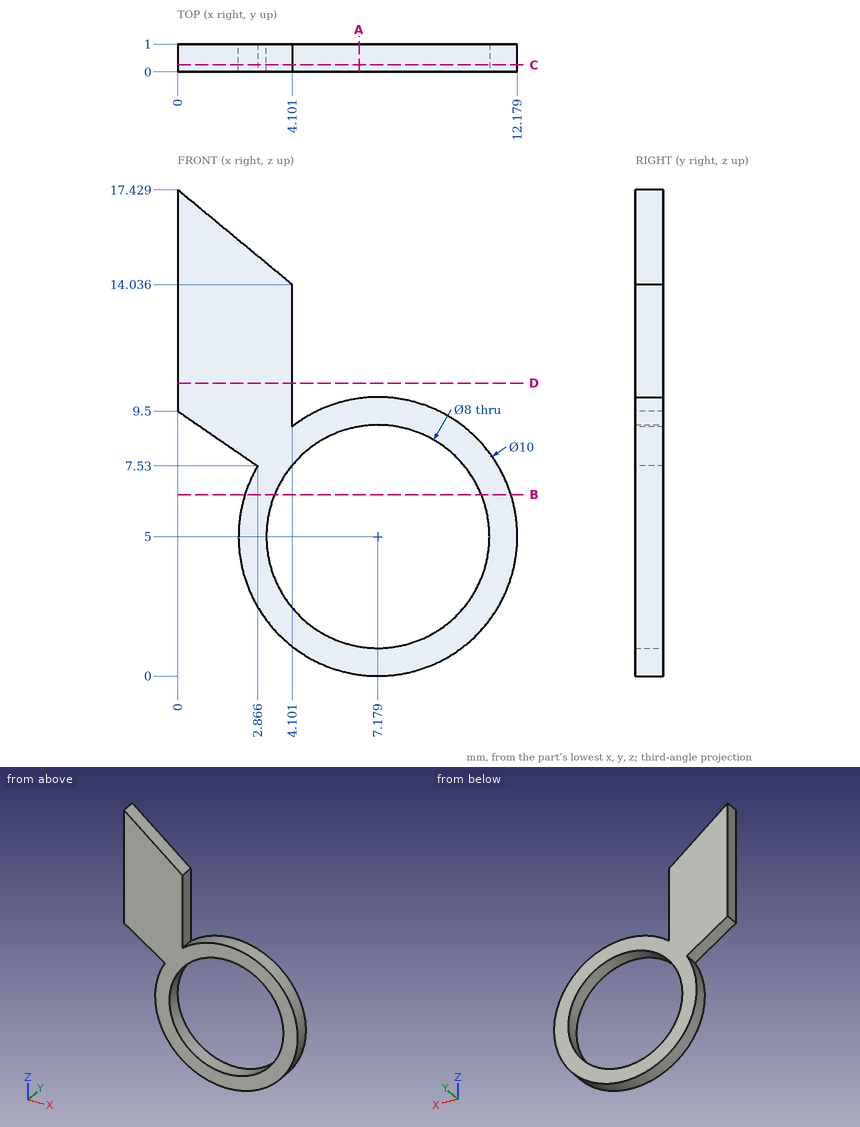
The drawing under review shows one solid part. Ordinate dimensions are in mm from its lowest x, y, z. Coordinates: 2 decimals unless noted, no trailing zeros. Order: outer loops, then holes, each group sorted by start corner. A loop starts at its lowest first (then second) coordinate and runs counter-clockwise, first axis right, second up. Notation, with made-up numbers: (-18, 22.5) - (-5, 22.5) arc R22 cw to (-5, 59.5) - close; hole circle Ø11 at (35, 78). An arc over 180 degrees is marked (long way). Put each result on its own line as item: value.
1) Take a section at D-D, the plane z = 10.5. Give the boundary of the cut face in (x, y).
Response values:
outline: (0, 0) - (4.1, 0) - (4.1, 1) - (0, 1) - close
2) Take a section at B-B, the plane z = 6.5. Give the boundary of the cut face in (x, y).
Response values:
outline: (2.41, 0) - (3.47, 0) - (3.47, 1) - (2.41, 1) - close; (10.89, 0) - (11.95, 0) - (11.95, 1) - (10.89, 1) - close
3) Insertion check: P1, Ø1, axis at x = 1.5, z = 5, coming from the +Y side. The pin has a flat end and moves straight along its axis. Give the tip position at first contact, or say it passes through.
Response values:
P1: passes through
4) Wall thickness on L1, parallel to Z at x = 7, y = 0.1; L2, parallel to Z at x = 4, y = 0.6; L3, parallel to X at y = 0.7, z = 2 (1 decimal): over which ranges is each line inside the solid? List them lowest first. Write a range as from..to.
Response values:
L1: z = 0..1, 9..10
L2: z = 1.14..2.57, 7.43..14.12
L3: x = 3.2..4.5, 9.8..11.2
5) Take a section at A-A, the plane x = 6.5. Give the boundary of the cut face in (y, z).
Response values:
outline: (0, 0.05) - (1, 0.05) - (1, 1.06) - (0, 1.06) - close; (0, 8.94) - (1, 8.94) - (1, 9.95) - (0, 9.95) - close
6) Take a section at C-C, the plane y = 0.25. Give the boundary of the cut face in (x, z) (1 decimal).
Response values:
outline: (0, 9.5) - (2.9, 7.5) arc R5 ccw (long way) to (4.1, 8.9) - (4.1, 14) - (0, 17.4) - close; hole circle Ø8 at (7.2, 5)
